CAD build for the part. Positions are in the model's coordinates, mm. A direction names the side the tool comes from. Give positions to 0.01 mm unless a question says otherwise; leave off trailing zeros. Order: outer loops, then holes, each group sorted by start corner. A loop starts at its lowest first (then second) coordinate and runs counter-clockwise, first axis right, second up. Notation, with made-up numbers: (44, 26.5) -> (74, 26.5) arc R12 cw to (74, 49.5) -> close; hole circle Ø2 at (-18, 84). An arc over 180 degrees is marked (long way). Use one line per item in the form item = value. Start each with the question number.
1) Drop flat-ended pins along their axis: P1, Ø2, axis at x = -2.5, z = -8, coming from the +Y side; P2, Ø5.5, axis at x = -2.5, z = -23.5, coming from the +Y side; P3, Ø1.5, axis at x = -7.5, y = -7, coming from the +Z side; P4, Ø2, axis at x = 4, y = -1.5, coming from the -Z side. Give the stop position or say it passes through.
2) Cut at C-C, the plane y = -6. Give the cut face in (x, z) (3 decimals).
3) Cut at D-D, the plane y = -3.25. Give the cut face in (x, z), and give its area (3 significant figures).
4) Probe line 1 (Z direction, x = -0.25, y = -6.75); line 2 (Z direction, x = 6.25, y = -7); line 3 (Y direction, x = 1.75, z = -12). List the from-to ranges inside material, lowest first.
5) Cut at A-A, the plane z = -25. Give the cut face in (x, y) (3 decimals).
6) Mould opens along Z. For faces 5 (the face through (-3.775, -4, 1)), 6 (the face through (0, -4, -13)), 7 (the face through (5.627, -4.437, 5.726)) say: pulls with the +Z half, pulls with the -Z half, needs draft (parallel to the pull), parting line crosses it, or undercut.
7) Cut at B-B, the plane x = 0. Give the cut face in (y, z) (3 decimals).
8) Tool access for faces 1 (the face through (0, -2, 0)), 2 (the face through (-6, -4, 2.5)), 3 (the face through (7.475, -4, 3)), 4 (the face through (6, -7, 0)): list every direction of +Z, -Z, +X, -X, +Y, -Y with a clear straight run to the whole face (end or side of a thin tool).
from build123d import *

# Parameters (mm, degrees)
F1_DEPTH       = 9
F2_W           = 18
F2_H           = 35
F3_DEPTH       = 5
F5_D           = 8.8
F5_DEPTH       = 10
F5_CBORE_D     = 14.25
F5_CBORE_DEPTH = 8
F5_TIP         = 2.6437867237


with BuildPart() as f1:
    # F0 (on Front) → F1 (new body)
    with BuildSketch(Plane.XZ):
        Polygon((-3.7746716016, 2.5), (-3.7746716016, 0), (3.7253283984, 0), (3.7253283984, 2.5), (7.4753283984, 2.5), (7.4753283984, 4), (3.7253283984, 7.5), (-3.7746716016, 7.5), (-7.5246716016, 4), (-7.5246716016, 2.5), align=None)
    extrude(amount=F1_DEPTH)

    # F2 (on face) → F3 (join)
    with BuildSketch(Plane.XZ.offset(9)):
        with Locations((0, -17.5)):
            Rectangle(F2_W, F2_H)
    extrude(amount=-F3_DEPTH)

    # F5
    with Locations(Plane.XZ.offset(9)):
        with Locations((0, -25)):
            CounterBoreHole(F5_D / 2, F5_CBORE_D / 2, F5_CBORE_DEPTH, depth=F5_DEPTH)
            with Locations((0, 0, -(F5_DEPTH + F5_TIP / 2))):  # 118° drill point
                Cone(0, F5_D / 2, F5_TIP, mode=Mode.SUBTRACT)


solid = f1.part
Result:
q1.P1 = -4
q1.P2 = through
q1.P3 = 4.72
q1.P4 = 0
q2.outline = (-9, -35) -> (9, -35) -> (9, 0) -> (3.725, 0) -> (3.725, 2.5) -> (7.475, 2.5) -> (7.475, 4) -> (3.725, 7.5) -> (-3.775, 7.5) -> (-7.525, 4) -> (-7.525, 2.5) -> (-3.775, 2.5) -> (-3.775, 0) -> (-9, 0) -> close; hole circle Ø14.25 at (0, -25)
q3.outline = (-7.52, 2.5) -> (-3.77, 2.5) -> (-3.77, 0) -> (3.73, 0) -> (3.73, 2.5) -> (7.48, 2.5) -> (7.48, 4) -> (3.73, 7.5) -> (-3.77, 7.5) -> (-7.52, 4) -> close
q3.area = 80.6 mm²
q4.line_1 = -35 to -32.12, -17.88 to 7.5
q4.line_2 = -35 to -28.42, -21.58 to 0, 2.5 to 5.14
q4.line_3 = -9 to -4
q5.outline = (-9, -9) -> (-7.125, -9) -> (-7.125, -4) -> (-9, -4) -> close; (7.125, -9) -> (9, -9) -> (9, -4) -> (7.125, -4) -> close
q6.face_5 = undercut
q6.face_6 = needs draft
q6.face_7 = pulls with the +Z half
q7.outline = (-9, -35) -> (-4, -35) -> (-4, -32.125) -> (-9, -32.125) -> close; (-9, -17.875) -> (-4, -17.875) -> (-4, 0) -> (0, 0) -> (0, 7.5) -> (-9, 7.5) -> close
q8.face_1 = -Z, +X, -X, +Y
q8.face_2 = -X, +Y, -Y
q8.face_3 = +Z, +X, +Y, -Y
q8.face_4 = +X, +Y, -Y
